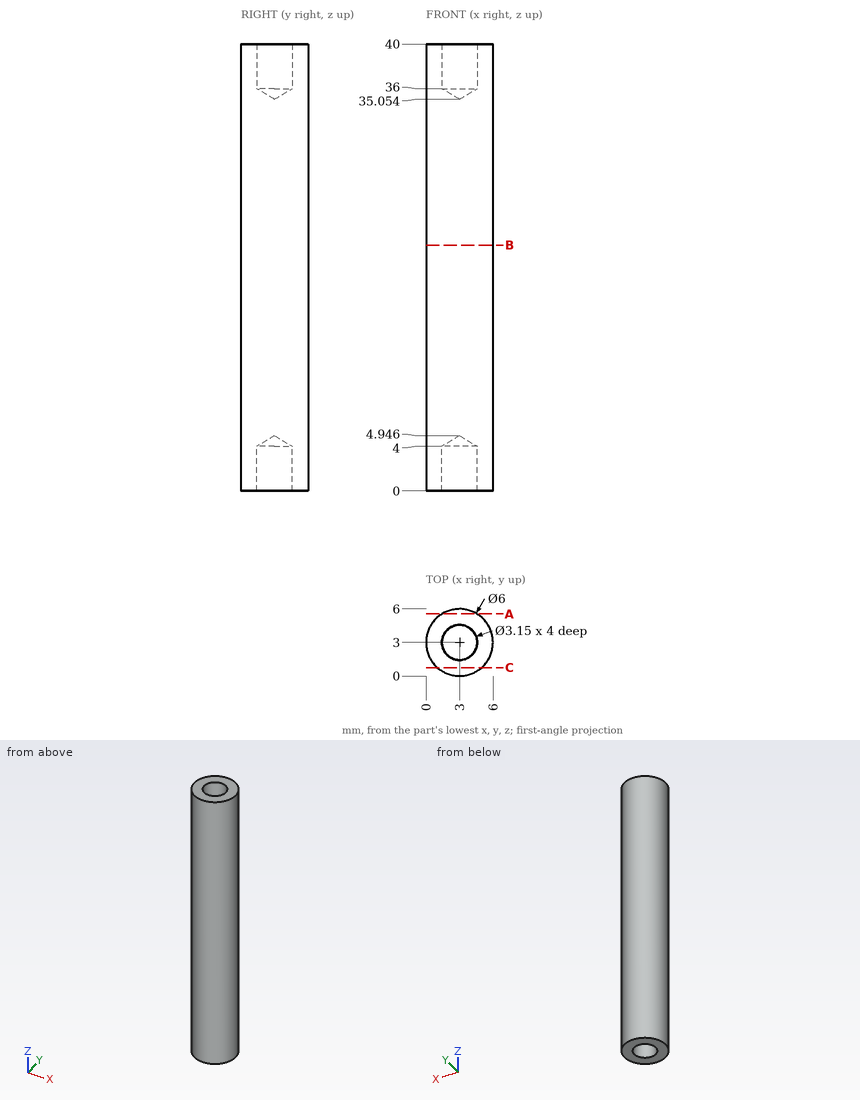
Check sheet for the drawn part. Datum: minimum x, y, z corner. Units: mm. Round coordinates to 2 decimals unless told otherwise and drop trailing zeros. Order: outer loops, then holes, each group sorted by start corner. A loop starts at its lowest first (then second) coordinate and runs counter-clockwise, first axis right, second up. Notation, with made-up numbers: (-26, -30) - (17, -30) arc R13 ccw to (17, -5) - close; hole circle Ø5 at (59.25, 80). An arc over 180 degrees is marked (long way). Use a Markdown table: item, result. Add a question column.
(1) Material ranges on line 1 along Y through (x, z) = (3, 2.6) (1 decimal); line 2 along Y through (x, z) = (2.9, 5); line 3 along Y through (x, z) = (2.05, 22) (1 decimal), recorded low to high. Write a range as [from, to].
(2) Sectioned sample at C-C, the plane y = 0.75. Enter the section's corners in (x, z) (1 decimal), and give its area (3 significant figures).
(3) Sectioned sample at A-A, the plane y = 5.55. Enter the section's corners in (x, z).
(4) Sectioned sample at B-B, the plane z = 22. Enter the section's corners in (x, y), and give its area (3 significant figures).
(5) Depth check by flat-ended pin: pin 1 (1 mm diameter, centred on y = 2, z = 33.5, fed in from +X); pin 2 (1.5 mm diameter, centred on x = 5.5, z = 14, fed in from -Y); pin 3 (2.5 mm diameter, centred on x = 3, y = 3, fed in from +Z) (1 decimal). Enter the tip coordinate at first touch or a pass-through.
Answers below:
| question | item | result |
|---|---|---|
| 1 | line 1 | [0, 1.4], [4.6, 6] |
| 1 | line 2 | [0, 6] |
| 1 | line 3 | [0.2, 5.8] |
| 2 | outline | (1, 0) - (5, 0) - (5, 40) - (1, 40) - close |
| 2 | area | 159 mm² |
| 3 | outline | (1.42, 0) - (4.58, 0) - (4.58, 40) - (1.42, 40) - close |
| 4 | outline | circle Ø6 at (3, 3) |
| 4 | area | 28.3 mm² |
| 5 | pin 1 | x = 5.96 |
| 5 | pin 2 | y = 0.56 |
| 5 | pin 3 | z = 35.8 |
